Can you work these out from the model? Positions are in its coordinate system, mm. Face numbers are marked on the shaded views. A direction names the side the tool comes from. Round coordinates to 2 decimals unless told otherwise and drop trailing zeros. Loops run counter-clockwise (first coordinate to the right, second up) from the corner with the lowest first, then second, coordinate; pieces in that order, holes last.
(1) Thinking about a two-plate mould opening in Y: for the marked faces 1, 2 and 3, which applies, released by +Y, released by -Y, zero draft, split by the parting line, or undercut?
(2) If I drill on line 1 along Y through (x, z) = (-7.5, 15); line 2 along X through (y, z) = (-20, 10); line 3 along Y through (x, z) = (-54, 17.25), over which ranges is the centre line in solid material (lowest first)?
(3) Which directions (+Z, -Z, +X, -X, +Y, -Y) give clear straight access to the entire face, cutting with the end or side of a thin tool? Please do the marked faces 4, 5 and 6.
(4) Will these pins go through, and if not, where does the flat tip stop? pin 1 Ø5.5 at (y, z) = (63, 9) entering from +X; pin 2 Ø4 at (y, z) = (-8, 2.5) entering from +X; pin 3 Ø7.5 at (x, z) = (2.5, 11.5) entering from -Y; pin 4 Ø12 at (x, y) = (-0.5, 57.5) entering from +Z.
(5) I want a section at B-B on z = 10.5. Give the number of separate pieces and of enclosed holes in the cut face, plus the area to 3 significant figures.
(6) I want a section at A-A on y = 61.5. Write out the boundary of the cut face in (x, z).
(7) I want a section at C-C on x = -2. Write out the boundary of the cut face in (y, z).
(8) I want a section at D-D on y = 9. Write out the boundary of the cut face in (x, z), plus the area to 3 significant figures.
from build123d import *

# Parameters (mm, degrees)
F0_R     = 50
F1_DEPTH = 3
F2_W     = 15.1
F2_H     = 15.1
F3_DEPTH = 3
F2_H_2   = 2
F2_W_2   = 2
F4_DEPTH = 18
F5_R     = 10


with BuildPart() as f1:
    # F0 (on Top) → F1 (new body)
    with BuildSketch(Plane.XY):
        Circle(F0_R)
    extrude(amount=F1_DEPTH)

    # F2 (on Top) → F3, piece 3 (join)
    with BuildSketch(Plane.XY):
        with BuildLine():
            ThreePointArc((-9.55, 49.0795018312), (-4.7971297897, 49.7693434333), (0, 50))
            Line((0, 50), (-7.55, 50))
            Line((-7.55, 50), (-9.55, 49.0795018312))
        make_face()
        with BuildLine():
            ThreePointArc((0, 50), (4.7971297897, 49.7693434333), (9.55, 49.0795018312))
            Line((9.55, 49.0795018312), (7.55, 50))
            Line((7.55, 50), (0, 50))
        make_face()
        with BuildLine():
            Line((47.0762701892, -18.4615082014), (47.2790953909, -16.2692083095))
            ThreePointArc((47.2790953909, -16.2692083095), (45.5000807553, -20.7302351954), (43.3012704728, -24.9999995088))
            Line((43.3012704728, -24.9999995088), (47.0762701892, -18.4615082014))
        make_face()
        with BuildLine():
            Line((39.5262701892, -31.5384917986), (43.3012704728, -24.9999995088))
            ThreePointArc((43.3012704728, -24.9999995088), (40.7029510127, -29.039107749), (37.7290953909, -32.8102935217))
            Line((37.7290953909, -32.8102935217), (39.5262701892, -31.5384917986))
        make_face()
        with BuildLine():
            ThreePointArc((-43.3012707255, -24.9999990711), (-45.5000808601, -20.7302349654), (-47.2790953909, -16.2692083095))
            Line((-47.2790953909, -16.2692083095), (-47.0762701892, -18.4615082014))
            Line((-47.0762701892, -18.4615082014), (-43.3012707255, -24.9999990711))
        make_face()
        with BuildLine():
            Line((-39.5262701892, -31.5384917986), (-37.7290953909, -32.8102935217))
            ThreePointArc((-37.7290953909, -32.8102935217), (-40.7029511595, -29.0391075432), (-43.3012707255, -24.9999990711))
            Line((-43.3012707255, -24.9999990711), (-39.5262701892, -31.5384917986))
        make_face()
    extrude(amount=F3_DEPTH)



with BuildPart() as f3:
    # F2 (on Top) → F3 (new body)
    with BuildSketch(Plane.XY):
        with Locations((0, 59.55)):
            Rectangle(F2_W, F2_H)
    extrude(amount=F3_DEPTH)


with BuildPart() as f3b:
    # F2 (on Top) → F3, piece 2 (new body)
    with BuildSketch(Plane.XY):
        Polygon((54.3353045939, -40.0884917986), (61.8853045939, -27.0115082014), (48.8083209968, -19.4615082014), (41.2583209968, -32.5384917986), align=None)
    extrude(amount=F3_DEPTH)


with BuildPart() as f3c:
    # F2 (on Top) → F3, piece 4 (new body)
    with BuildSketch(Plane.XY):
        Polygon((-48.8083209968, -19.4615082014), (-61.8853045939, -27.0115082014), (-54.3353045939, -40.0884917986), (-41.2583209968, -32.5384917986), align=None)
    extrude(amount=F3_DEPTH)


with BuildPart() as f1_1:
    add(f1.part)

    add(f3.part)  # F4 merges F3

    add(f3b.part)  # F4 merges F3b

    add(f3c.part)  # F4 merges F3c
    # F2 (on Top) → F4 (join)
    with BuildSketch(Plane.XY):
        Polygon((-47.0762701892, -18.4615082014), (-47.2790953909, -16.2692083095), (-62.8853045939, -25.2794573939), (-61.8853045939, -27.0115082014), (-48.8083209968, -19.4615082014), align=None)
        Polygon((-39.5262701892, -31.5384917986), (-43.3012707255, -24.9999990711), (-47.0762701892, -18.4615082014), (-48.8083209968, -19.4615082014), (-41.2583209968, -32.5384917986), align=None)
        Polygon((-53.3353045939, -41.8205426061), (-37.7290953909, -32.8102935217), (-39.5262701892, -31.5384917986), (-41.2583209968, -32.5384917986), (-54.3353045939, -40.0884917986), align=None)
        Polygon((-54.3353045939, -40.0884917986), (-61.8853045939, -27.0115082014), (-63.6173554015, -28.0115082014), (-56.0673554015, -41.0884917986), align=None)
        Polygon((-61.8853045939, -27.0115082014), (-62.8853045939, -25.2794573939), (-64.6173554015, -26.2794573939), (-63.6173554015, -28.0115082014), align=None)
        Polygon((-55.0673554015, -42.8205426061), (-53.3353045939, -41.8205426061), (-54.3353045939, -40.0884917986), (-56.0673554015, -41.0884917986), align=None)
        Polygon((47.0762701892, -18.4615082014), (43.3012704728, -24.9999995088), (39.5262701892, -31.5384917986), (41.2583209968, -32.5384917986), (48.8083209968, -19.4615082014), align=None)
        Polygon((62.8853045939, -25.2794573939), (47.2790953909, -16.2692083095), (47.0762701892, -18.4615082014), (48.8083209968, -19.4615082014), (61.8853045939, -27.0115082014), align=None)
        Polygon((64.6173554015, -26.2794573939), (62.8853045939, -25.2794573939), (61.8853045939, -27.0115082014), (63.6173554015, -28.0115082014), align=None)
        Polygon((63.6173554015, -28.0115082014), (61.8853045939, -27.0115082014), (54.3353045939, -40.0884917986), (56.0673554015, -41.0884917986), align=None)
        Polygon((54.3353045939, -40.0884917986), (53.3353045939, -41.8205426061), (55.0673554015, -42.8205426061), (56.0673554015, -41.0884917986), align=None)
        Polygon((39.5262701892, -31.5384917986), (37.7290953909, -32.8102935217), (53.3353045939, -41.8205426061), (54.3353045939, -40.0884917986), (41.2583209968, -32.5384917986), align=None)
        with Locations((0, 68.1)):
            Rectangle(F2_W, F2_H_2)
        with Locations((-8.55, 68.1)):
            Rectangle(F2_W_2, F2_H_2)
        with Locations((8.55, 68.1)):
            Rectangle(F2_W_2, F2_H_2)
        Polygon((7.55, 50), (9.55, 49.0795018312), (9.55, 67.1), (7.55, 67.1), (7.55, 52), align=None)
        Polygon((-9.55, 67.1), (-9.55, 49.0795018312), (-7.55, 50), (-7.55, 52), (-7.55, 67.1), align=None)
        Polygon((-7.55, 50), (0, 50), (7.55, 50), (7.55, 52), (-7.55, 52), align=None)
    extrude(amount=F4_DEPTH)

    # F5
    f5_edges = [f1_1.edges().sort_by_distance(p)[0] for p in [
        (-9.55, 49.079502, 1.5),
        (9.55, 49.079502, 1.5),
        (-47.279095, -16.269208, 1.5),
        (-37.729095, -32.810294, 1.5),
        (37.729095, -32.810294, 1.5),
        (47.279095, -16.269208, 1.5),
    ]]
    fillet(f5_edges, radius=F5_R)


solid = f1_1.part
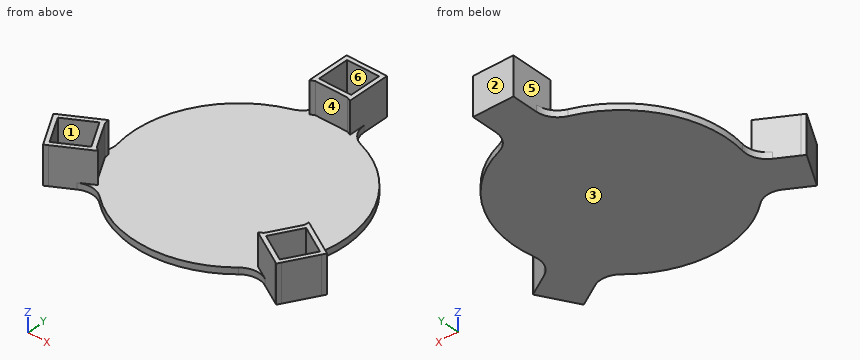
Filled sheet:
1. face 1: undercut
1. face 2: released by +Y
1. face 3: zero draft
2. line 1: y = 50 to 52, 67.1 to 69.1
2. line 2: x = -53.74 to -49.74, -48.5 to -46.19, 46.19 to 48.5, 49.74 to 53.74
2. line 3: y = -42.2 to -39.89, -22.46 to -20.15
3. face 4: +Z, -Y
3. face 5: +Z, -X, +Y
3. face 6: +Z
4. pin 1: stops at x = 9.55
4. pin 2: stops at x = 49.64
4. pin 3: stops at y = 50
4. pin 4: stops at z = 18
5. separate pieces: 3
5. enclosed holes: 3
5. area: 416 mm2
6. outline: (-9.55, 0) - (9.55, 0) - (9.55, 18) - (7.55, 18) - (7.55, 3) - (-7.55, 3) - (-7.55, 18) - (-9.55, 18) - close
7. outline: (-49.96, 0) - (69.1, 0) - (69.1, 18) - (67.1, 18) - (67.1, 3) - (52, 3) - (52, 18) - (50, 18) - (50, 3) - (-49.96, 3) - close
8. outline: (-49.18, 0) - (49.18, 0) - (49.18, 3) - (-49.18, 3) - close
8. area: 295 mm2
